Could you check a few things on this model? Use its own coordinates, in mm. Face numbers are marked on the shaded views. A direction names the side the tool comes from. Give positions to 0.01 mm unless a question says otherwise; leave off trailing zeros. Loops run counter-clockwise (first coordinate to the right, second up) from the corner with the lowest first, then second, coordinate; pieces in that order, holes last. Notation, with made-up numbers: M -22.75,65.25 L 35.25,65.25 A29 ccw 35.25,98.25 Z; hole C 67.25,45.25 d3. An arc over 180 degrees is marked long. Write each question's results on one line, items separated by ' | '. Start each with the question number.
from build123d import *

# Parameters (mm, degrees)
BOSS_EXTRUDE1_DEPTH      = 2.3476
BOSS_EXTRUDE1_DEPTH_BACK = 4.293
CUT_EXTRUDE1_DEPTH       = 32.505304994
SKETCH3_R                = 1.575
CUT_EXTRUDE2_DEPTH       = 2.593
SKETCH4_R                = 1
CUT_EXTRUDE3_DEPTH       = 36.667872697


with BuildPart() as part:
    # Sketch1 → Boss-Extrude1 (new, two sides: drawn at the far end of the back side and taken through both)
    with BuildSketch(Plane.XY.offset(-BOSS_EXTRUDE1_DEPTH_BACK)):
        with BuildLine():
            Line((10.3124, -8.55), (22.8124, -8.55))
            ThreePointArc((22.8124, -8.55), (28.8124, -14.55), (22.8124, -20.55))
            Line((22.8124, -20.55), (10.3124, -20.55))
            ThreePointArc((10.3124, -20.55), (4.3124, -14.55), (10.3124, -8.55))
        make_face()
    extrude(amount=BOSS_EXTRUDE1_DEPTH + BOSS_EXTRUDE1_DEPTH_BACK)

    # Sketch2 → Cut-Extrude1 (cut, through all)
    with BuildSketch(Plane.XZ.offset(20.55)):
        with BuildLine():
            Line((4.3124, 0.15), (20.65, 0.15))
            ThreePointArc((20.65, 0.15), (21.575, -0.775), (20.65, -1.7))
            Line((20.65, -1.7), (4.3124, -1.7))
            ThreePointArc((4.3124, -1.7), (3.3874, -0.775), (4.3124, 0.15))
        make_face()
    extrude(amount=-CUT_EXTRUDE1_DEPTH, mode=Mode.SUBTRACT)

    # Sketch3 → Cut-Extrude2 (cut)
    with BuildSketch(Plane(origin=(0, 0, -4.293), x_dir=(-1, 0, 0), z_dir=(0, 0, -1))):
        with Locations((-10.3124, -14.55)):
            Circle(SKETCH3_R)
    extrude(amount=-CUT_EXTRUDE2_DEPTH, mode=Mode.SUBTRACT)

    # Sketch4 → Cut-Extrude3 (cut, through all)
    with BuildSketch(Plane(origin=(0, 0, 0.15), x_dir=(-1, 0, 0), z_dir=(0, 0, -1))):
        with Locations((-10.3124, -14.55)):
            Circle(SKETCH4_R)
    extrude(amount=-CUT_EXTRUDE3_DEPTH, mode=Mode.SUBTRACT)


solid = part.part
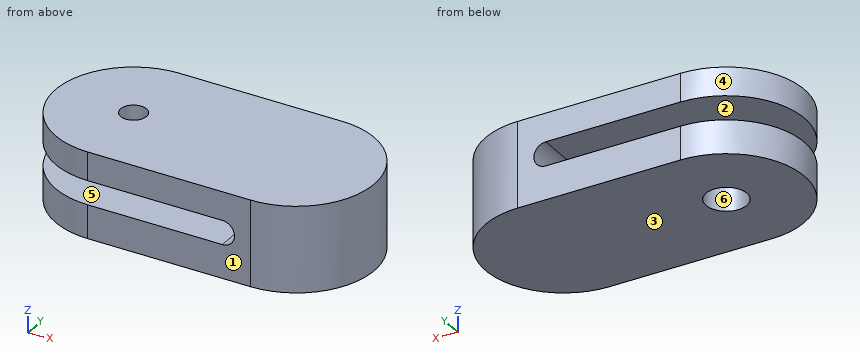
1) Thinking about a two-plate mould opening in Z: for the marked faces 1, 2 and 3, which applies, pulls with the +Z half, pulls with the -Z half, needs draft (parallel to the pull), parting line crosses it, or undercut?
2) Which directions (+Z, -Z, +X, -X, +Y, -Y) give clear straight access to the entire face, cutting with the end or side of a thin tool? Please do the marked faces 4, 5 and 6.
3) Please list where these lines run through material, in increasing order: line 1 (Z direction, x = 7.75, y = -19.75); line 2 (Y direction, x = 10.5, z = -2.5); line 3 (X direction, y = -15, z = -1.25). Write a range as from..to.
4) I'm going to push flat-ended pins straight in: P1, Ø3, axis at x = 10.5, y = -14.5, coming from the +Z side; P2, Ø1.6, axis at x = 10.31, y = -14.55, coming from the -Z side; P3, Ø1.5, axis at y = -18, z = 1.5, coming from the +X side. Where does each tip first touch, or does it pass through?
5) If we section it at C-C on z = 1: Write out the boundary of the cut face in (x, y), plus the area to 3 significant figures.
6) If we section it at A-A on y = -14.55: Write out the boundary of the cut face in (x, z) (3 decimals), plus the area to 3 significant figures.
7) If we section it at B-B on x = 13.75: Write out the boundary of the cut face in (y, z), plus the area to 3 significant figures.
8) If we section it at D-D on y = -13.25: Write out the boundary of the cut face in (x, z) (3 decimals), plus the area to 3 significant figures.
Calculated:
1) face 1: needs draft | face 2: undercut | face 3: pulls with the -Z half
2) face 4: +Z, -Z, -X | face 5: -X, +Y, -Y | face 6: -Z
3) line 1: z = -4.29..-1.7, 0.15..2.35 | line 2: y = -20.55..-16.11, -12.99..-8.55 | line 3: x = 21.44..28.8
4) P1: stops at z = 2.35 | P2: passes through | P3: stops at x = 28.17
5) outline: M 10.31,-20.55 L 22.81,-20.55 A6 ccw 22.81,-8.55 L 10.31,-8.55 A6 ccw Z; hole C 10.31,-14.55 d2 | area: 260 mm2
6) outline: M 4.312,-4.293 L 8.737,-4.293 L 8.737,-1.7 L 4.312,-1.7 Z; M 4.312,0.15 L 9.312,0.15 L 9.312,2.348 L 4.312,2.348 Z; M 11.312,0.15 L 20.65,0.15 A0.925 cw 20.65,-1.7 L 11.887,-1.7 L 11.887,-4.293 L 28.812,-4.293 L 28.812,2.348 L 11.312,2.348 Z | area: 119 mm2
7) outline: M -20.55,-4.29 L -8.55,-4.29 L -8.55,-1.7 L -20.55,-1.7 Z; M -20.55,0.15 L -8.55,0.15 L -8.55,2.35 L -20.55,2.35 Z | area: 57.5 mm2
8) outline: M 4.455,-4.293 L 9.423,-4.293 L 9.423,-1.7 L 4.455,-1.7 Z; M 4.455,0.15 L 20.65,0.15 A0.925 cw 20.65,-1.7 L 11.202,-1.7 L 11.202,-4.293 L 28.67,-4.293 L 28.67,2.348 L 4.455,2.348 Z | area: 125 mm2
